Here's how the part is built. I have some questions about the finished solid (model axes, mm). A direction names the side the tool comes from. Coordinates: 2 decimals unless noted, no trailing zeros. Loops run counter-clockwise (first coordinate to the right, second up) from the corner with the lowest first, then second, coordinate; pieces in that order, holes last.
from build123d import *

# Parameters (mm, degrees)
F1_DEPTH = 25
F0_R     = 35
F2_DEPTH = 5
F3_DEPTH = 2.5
F4_DEPTH = 2.5


with BuildPart() as f1:
    # F0 (on Top) → F1 (new body)
    with BuildSketch(Plane.XY):
        with BuildLine():
            ThreePointArc((32.169506, 23.772314), (37.991974, 12.514387), (40, 0))
            ThreePointArc((40, 0), (37.991974, -12.514387), (32.169506, -23.772314))
            ThreePointArc((32.169506, -23.772314), (65.028774, 0), (32.169506, 23.772314))
        make_face()
        with BuildLine():
            ThreePointArc((36.233804, 22.211741), (62.528774, 0), (36.233804, -22.211741))
            ThreePointArc((36.233804, -22.211741), (42.5, 0), (36.233804, 22.211741))
        make_face(mode=Mode.SUBTRACT)
    extrude(amount=F1_DEPTH)

    # F0 (on Top) → F2 (join)
    with BuildSketch(Plane.XY):
        with BuildLine():
            ThreePointArc((32.169506, -23.772314), (37.991974, -12.514387), (40, 0))
            ThreePointArc((40, 0), (37.991974, 12.514387), (32.169506, 23.772314))
            ThreePointArc((32.169506, 23.772314), (-40, 0), (32.169506, -23.772314))
        make_face()
        Circle(F0_R, mode=Mode.SUBTRACT)
    extrude(amount=F2_DEPTH)

    # F0 (on Top) → F3 (join)
    with BuildSketch(Plane.XY):
        Circle(F0_R)
    extrude(amount=F3_DEPTH)

    # F0 (on Top) → F4 (join)
    with BuildSketch(Plane.XY):
        with BuildLine():
            ThreePointArc((36.233804, 22.211741), (42.5, 0), (36.233804, -22.211741))
            ThreePointArc((36.233804, -22.211741), (62.528774, 0), (36.233804, 22.211741))
        make_face()
    extrude(amount=F4_DEPTH)


solid = f1.part
Q1. We'd pull the mould along Y, two halves only. Please class faces 4 (the cylindrical face through (-39.975, 1.403, 2.465)), 5 (the flat face through (0, 0, 2.5)), 6 (the flat face through (42, 0, 25)): pulls with the +Y half, pulls with the -Y half, needs draft (parallel to the pull), parting line crosses it, or undercut.
Q2. Suppose I cut it at C-C on y = 27.5. Write out the boundary of the cut face in (x, z), and give its area (3 significant figures).
Q3. Suppose I cut it at D-D on x = 38.5. Write out the boundary of the cut face in (y, z), and give its area (3 significant figures).
Q4. For faces 1 (the cylindrical face through (-28, -21, 4)), 2 (the flat face through (12, 1, 0)), 3 (the flat face through (-0.2, -35.4, 5)), which set-ups out of +Z, -Z, +X, -X, +Y, -Y let a thin tool reach every point of the face, with its end or its side?
Q5. Will these pins go through, and if not, where does the flat tip stop? P1, Ø13, axis at x = 46.5, y = -7, coming from the +Z side; P2, Ø5, axis at x = 52.5, z = 17, coming from the -Y side; P3, Ø12, axis at x = -12.5, y = 13, coming from the +Z side; P4, Ø10, axis at y = 6.5, z = 6.5, coming from the +X side.
Q6. Please list where these lines run through material, in increasing order: probe 1 along Y at (x, z) = (0, 4.4); probe 2 along X at (y, z) = (3, 3.75); probe 3 along Z at (x, y) = (0.5, 26).
Q7. Suppose I cut it at A-A on z = 17.25. Write out the boundary of the cut face in (x, y), and give its area (3 significant figures).
Q8. Suppose I cut it at B-B on x = 0. Write out the boundary of the cut face in (y, z), and give its area (3 significant figures).
Check values:
1. face 4: parting line crosses it
1. face 5: undercut
1. face 6: needs draft
2. outline: (-29.05, 0) - (29.05, 0) - (29.05, 5) - (21.65, 5) - (21.65, 2.5) - (-21.65, 2.5) - (-21.65, 5) - (-29.05, 5) - close
2. area: 182 mm2
3. outline: (-24.98, 0) - (24.98, 0) - (24.98, 25) - (22.48, 25) - (22.48, 2.5) - (18, 2.5) - (18, 25) - (10.85, 25) - (10.85, 5) - (-10.85, 5) - (-10.85, 25) - (-18, 25) - (-18, 2.5) - (-22.48, 2.5) - (-22.48, 25) - (-24.98, 25) - close
3. area: 614 mm2
4. face 1: +Z
4. face 2: -Z, +X, -X, +Y, -Y
4. face 3: +Z, -X
5. P1: stops at z = 25
5. P2: stops at y = -22.94
5. P3: stops at z = 2.5
5. P4: stops at x = 64.98
6. probe 1: y = -40 to -35, 35 to 40
6. probe 2: x = -39.89 to -34.87, 34.87 to 42.39, 62.33 to 64.85
6. probe 3: z = 0 to 2.5
7. outline: (32.17, -23.77) arc R25.03 ccw (long way) to (32.17, 23.77) arc R40 cw to (40, 0) arc R40 cw to start; hole (36.23, -22.21) arc R22.53 ccw (long way) to (36.23, 22.21) arc R42.5 cw to start
7. area: 338 mm2
8. outline: (-40, 0) - (40, 0) - (40, 5) - (35, 5) - (35, 2.5) - (-35, 2.5) - (-35, 5) - (-40, 5) - close
8. area: 225 mm2
